Design review of the part shown in the three views and the two pictorial views. Dimensions are in mm from the part's minimum x, y and z. Coordinates: 2 decimals unless noted, no trailing zeros. Write each loop counter-clockwise with the first axis right and the second up, starting at its lowest first coordinate (ties: lowest second). Pieces come first, ordered by that corner, then holes. Notation, with made-up numbers: (47, 45.5) - (83, 45.5) arc R28 cw to (83, 78.5) - close; hole circle Ø11 at (85, 83). An arc over 180 degrees is marked (long way). Return JSON: item names as keys, results as strings. Group by question number.
(1) We need section B-B on x = 3.81. State the section outline as (y, z) points.
(2) We need section A-A on y = 29.21. State the section outline as (x, z) points.
(3) We need section C-C on z = 0.3. State the section outline as (x, y) points (1 decimal).
(4) To check wall thickness, follow L1, parallel to Y at x = 3.81, z = 1; L2, parallel to Y at x = 5, z = 1.5; L3, parallel to X at y = 1, z = 0.2. State the ranges of each line that lie inside material, in increasing order. Write a range as from..to.
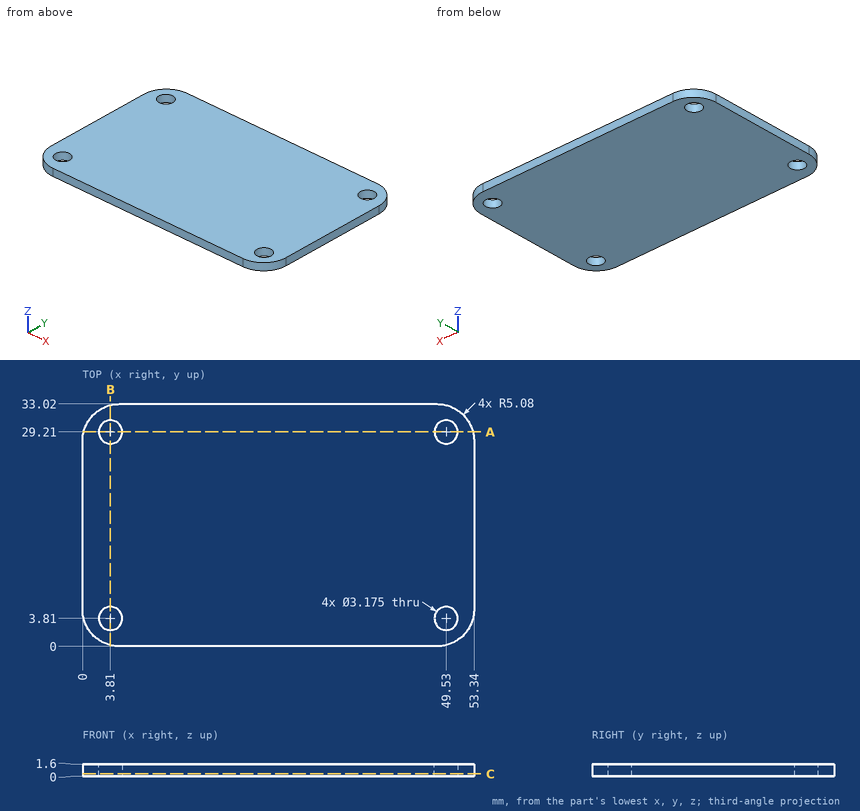
Ans:
{
 "1": {"outline": "(0.16, 0) - (2.22, 0) - (2.22, 1.6) - (0.16, 1.6) - close; (5.4, 0) - (27.62, 0) - (27.62, 1.6) - (5.4, 1.6) - close; (30.8, 0) - (32.86, 0) - (32.86, 1.6) - (30.8, 1.6) - close"},
 "2": {"outline": "(0.16, 0) - (2.22, 0) - (2.22, 1.6) - (0.16, 1.6) - close; (5.4, 0) - (47.94, 0) - (47.94, 1.6) - (5.4, 1.6) - close; (51.12, 0) - (53.18, 0) - (53.18, 1.6) - (51.12, 1.6) - close"},
 "3": {"outline": "(0, 5.1) arc R5.1 ccw to (5.1, 0) - (48.3, 0) arc R5.1 ccw to (53.3, 5.1) - (53.3, 27.9) arc R5.1 ccw to (48.3, 33) - (5.1, 33) arc R5.1 ccw to (0, 27.9) - close; hole circle Ø3.2 at (3.8, 3.8); hole circle Ø3.2 at (3.8, 29.2); hole circle Ø3.2 at (49.5, 3.8); hole circle Ø3.2 at (49.5, 29.2)"},
 "4": {"L1": "0.16..2.22, 5.4..27.62, 30.8..32.86", "L2": "0..2.76, 4.86..28.16, 30.26..33.02", "L3": "2.05..51.29"}
}
